Part model, mm, in its own coordinate system. Coordinates: 2 decimals unless noted, no trailing zeros. Write each loop counter-clockwise with the first axis right and the second up, starting at its lowest first coordinate (ties: lowest second). Pieces come first, ordered by that corner, then holes. Notation, with made-up numbers: (19.5, 81.25) -> (50.5, 81.25) arc R28 ccw to (50.5, 109.25) -> close; hole circle Ø7 at (-7.75, 7). An arc over 180 degrees is marked (long way). Write item = value, one per line.
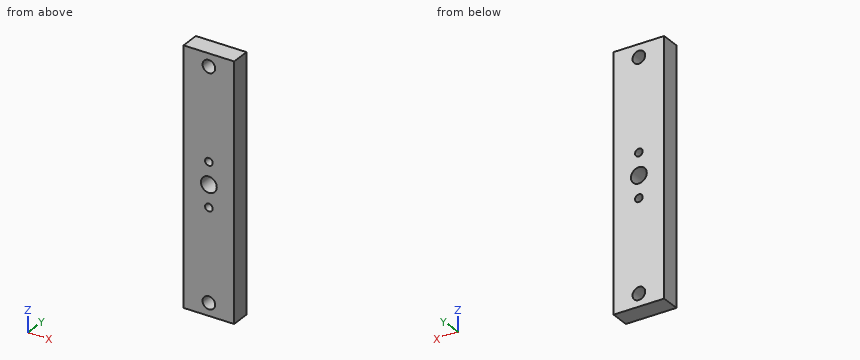
from build123d import *

# Parameters (mm, degrees)
SKETCH1_W                          = 25.4
SKETCH1_H                          = 9.525
EXTRUDE1_DEPTH                     = 127
F_1_4_0_25_DIAMETER_HOLE1_D        = 6.35
F_1_4_0_25_DIAMETER_HOLE1_DEPTH    = 12.7
F_1_4_0_25_DIAMETER_HOLE1_TIP      = 1.907732465
F_5_16_0_3125_DIAMETER_HOLE1_D     = 7.9375
F_5_16_0_3125_DIAMETER_HOLE1_DEPTH = 12.7
F_5_16_0_3125_DIAMETER_HOLE1_TIP   = 2.384665582
CIRPATTERN1_COUNT                  = 2


with BuildPart() as part:
    # Sketch1 → Extrude1 (new body)
    with BuildSketch(Plane.XY):
        Rectangle(SKETCH1_W, SKETCH1_H)
    extrude(amount=EXTRUDE1_DEPTH)

    # 1/4 (0.25) Diameter Hole1
    with Locations(Plane(origin=(0, 4.7625, 6.35), x_dir=(0, 0, 1), z_dir=(0, 1, 0))):
        with Locations((0, 0), (114.3, 0)):
            Hole(F_1_4_0_25_DIAMETER_HOLE1_D / 2, depth=F_1_4_0_25_DIAMETER_HOLE1_DEPTH)
            with Locations((0, 0, -(F_1_4_0_25_DIAMETER_HOLE1_DEPTH + F_1_4_0_25_DIAMETER_HOLE1_TIP / 2))):  # 118° drill point
                Cone(0, F_1_4_0_25_DIAMETER_HOLE1_D / 2, F_1_4_0_25_DIAMETER_HOLE1_TIP, mode=Mode.SUBTRACT)

    # 5/16 (0.3125) Diameter Hole1
    with Locations(Plane(origin=(0, 4.7625, 63.5), x_dir=(0, 0, 1), z_dir=(0, 1, 0))):
        with Locations((0, 0)):
            Hole(F_5_16_0_3125_DIAMETER_HOLE1_D / 2, depth=F_5_16_0_3125_DIAMETER_HOLE1_DEPTH)
            with Locations((0, 0, -(F_5_16_0_3125_DIAMETER_HOLE1_DEPTH + F_5_16_0_3125_DIAMETER_HOLE1_TIP / 2))):  # 118° drill point
                Cone(0, F_5_16_0_3125_DIAMETER_HOLE1_D / 2, F_5_16_0_3125_DIAMETER_HOLE1_TIP, mode=Mode.SUBTRACT)

    # Sketch6 → #25 (0.1495) Diameter Hole1 (revolve, cut)
    with BuildSketch(Plane(origin=(0, 4.7625, 74.549), x_dir=(0, 0, 1), z_dir=(1, 0, 0))):
        Polygon((0, 0), (0, 13.840824014), (1.89865, 12.7), (1.89865, 0), align=None)
    f_25_0_1495_diameter_hole1 = revolve(axis=Axis((0, 11.1125, 74.549), (0, -1, 0)), mode=Mode.SUBTRACT)

    # CirPattern1: #25 (0.1495) Diameter Hole1 ×2 about axis
    cirpattern1_axis = Axis((0, 0, 63.5), (0, 1, 0))
    for i in range(1, CIRPATTERN1_COUNT):
        add(f_25_0_1495_diameter_hole1.rotate(cirpattern1_axis, i * 360 / CIRPATTERN1_COUNT), mode=Mode.SUBTRACT)


solid = part.part
Q1. Probe line 1 (X direction, y = 2.5, z = 52.5); line 2 (Z direction, x = 2.5, y = -1.75); line 3 (X direction, y = -2.5, z = 63.5). List the from-to ranges inside material, lowest first. Write a range as from..to.
Model answer:
line_1 = -12.7..-1.9, 1.9..12.7
line_2 = 0..4.39, 8.31..60.42, 66.58..118.69, 122.61..127
line_3 = -12.7..-3.97, 3.97..12.7
Q2. Saw through at C-C on y = -1.5. Count the separate pieces of the cut face and the enclosed holes in it, and give its area (3 significant figures).
Model answer:
separate_pieces = 1
enclosed_holes = 5
area = 3,090 mm²
Q3. Saw through at B-B on z = 120.65. Give the cut face in (x, y) (1 decimal).
Model answer:
outline = (-12.7, -4.8) -> (-3.2, -4.8) -> (-3.2, 4.8) -> (-12.7, 4.8) -> close; (3.2, -4.8) -> (12.7, -4.8) -> (12.7, 4.8) -> (3.2, 4.8) -> close
Q4. Saw through at A-A on x = 0. Give the cut face in (y, z) (1 decimal), and give its area (3 significant figures).
Model answer:
outline = (-4.8, 0) -> (4.8, 0) -> (4.8, 3.2) -> (-4.8, 3.2) -> close; (-4.8, 9.5) -> (4.8, 9.5) -> (4.8, 50.6) -> (-4.8, 50.6) -> close; (-4.8, 54.3) -> (4.8, 54.3) -> (4.8, 59.5) -> (-4.8, 59.5) -> close; (-4.8, 67.5) -> (4.8, 67.5) -> (4.8, 72.7) -> (-4.8, 72.7) -> close; (-4.8, 76.4) -> (4.8, 76.4) -> (4.8, 117.5) -> (-4.8, 117.5) -> close; (-4.8, 123.8) -> (4.8, 123.8) -> (4.8, 127) -> (-4.8, 127) -> close
area = 941 mm²
Q5. Pin check, flat tip, straight feed: pin 1 (8.5 mm diameter, centred on x = 0, z = 120.65, fed in from -Y). Stop position of the tip, or through.
Model answer:
pin_1 = -4.76
Q6. Saw through at D-D on z = 63.5. Give the cut face in (x, y).
Model answer:
outline = (-12.7, -4.76) -> (-3.97, -4.76) -> (-3.97, 4.76) -> (-12.7, 4.76) -> close; (3.97, -4.76) -> (12.7, -4.76) -> (12.7, 4.76) -> (3.97, 4.76) -> close
